Read the model definition and answer for the solid it produces. Units are mm, in the model's axes. A direction names the side the tool comes from. Coordinates: 2 decimals unless noted, no trailing zeros. Order: outer loops, then holes, each group sorted by start corner. A loop starts at its lowest first (then second) coordinate and runs counter-clockwise, first axis right, second up. Notation, with made-up numbers: (-22.5, 3.25) -> (34.5, 3.25) arc R15 cw to (34.5, 12.25) -> close; hole circle Ø11 at (34.25, 55). An arc over 180 degrees is marked (long way). Answer in a Markdown table with one row per item.
from build123d import *

# Parameters (mm, degrees)
SKETCH1_W           = 30
SKETCH1_H           = 10
SKETCH1_R           = 1.75
BOSS_EXTRUDE1_DEPTH = 1
SKETCH2_W           = 30
SKETCH2_H           = 2.5
BOSS_EXTRUDE2_DEPTH = 10
CHAMFER1_SIZE       = 2
CHAMFER1_SIZE2      = 9.409260219


with BuildPart() as part:
    # Sketch1 → Boss-Extrude1 (new body)
    with BuildSketch(Plane.XY):
        Rectangle(SKETCH1_W, SKETCH1_H)
        with Locations((-10, 0.2)):
            Circle(SKETCH1_R, mode=Mode.SUBTRACT)
        with Locations((10, 0.2)):
            Circle(SKETCH1_R, mode=Mode.SUBTRACT)
    extrude(amount=BOSS_EXTRUDE1_DEPTH)

    # Sketch2 → Boss-Extrude2 (add)
    with BuildSketch(Plane.XY):
        with Locations((0, -6.25)):
            Rectangle(SKETCH2_W, SKETCH2_H)
    extrude(amount=BOSS_EXTRUDE2_DEPTH)

    # Chamfer1
    chamfer1_edges = [part.edges().sort_by_distance(p)[0] for p in [
        (0, -7.5, 10),
    ]]
    chamfer1_side = [part.faces().sort_by_distance(p)[0] for p in [
        (0, -6.25, 10),
    ]]
    chamfer(chamfer1_edges, length=CHAMFER1_SIZE, length2=CHAMFER1_SIZE2, reference=chamfer1_side[0])


solid = part.part
Q1. The part is cut by section D-D (y = -2.75). Write down the section's boundary in (x, z), then the cut area to 3 significant figures.
Outcome:
| item | result |
|---|---|
| outline | (-15, 0) -> (15, 0) -> (15, 1) -> (-15, 1) -> close |
| area | 30.0 mm² |
Q2. For a pull along Y with two mould halves and no side action, classify faces 3 (the face through (0, -5, 5)), 4 (the face through (11.669, 0.726, 0.493)), 5 (the face through (0, -1, 0)) as pulls with the +Y half, pulls with the -Y half, needs draft (parallel to the pull), parting line crosses it, or undercut.
Outcome:
| item | result |
|---|---|
| face 3 | pulls with the +Y half |
| face 4 | undercut |
| face 5 | needs draft |
Q3. For faces 1 (the face through (-8.331, 0.726, 0.493)), 2 (the face through (0, 0, 1)), determine the directions among +Z, -Z, +X, -X, +Y, -Y from which every point of the face is accessible in a straight line to the end or side of a thin tool.
Outcome:
| item | result |
|---|---|
| face 1 | +Z, -Z |
| face 2 | +Z, +X, -X, +Y |
Q4. The part is cut by section C-C (x = -5). Write down the section's boundary in (y, z).
Outcome:
| item | result |
|---|---|
| outline | (-7.5, 0) -> (5, 0) -> (5, 1) -> (-5, 1) -> (-5, 10) -> (-5.5, 10) -> (-7.5, 0.59) -> close |
Q5. The part is cut by section A-A (x = -10). Write down the section's boundary in (y, z), then the cut area to 3 significant figures.
Outcome:
| item | result |
|---|---|
| outline | (-7.5, 0) -> (-1.55, 0) -> (-1.55, 1) -> (-5, 1) -> (-5, 10) -> (-5.5, 10) -> (-7.5, 0.59) -> close; (1.95, 0) -> (5, 0) -> (5, 1) -> (1.95, 1) -> close |
| area | 22.1 mm² |
Q6. Given pin 1 (2.5 mm diameter, centred on x = 2, z = 7, fed in from +Y); pin 2 (5 mm diameter, centred on x = 4.5, y = -1, fed in from +Z); pin 3 (6 mm diameter, centred on x = 2, z = 7.5, fed in from -Y), each flat-ended and moving along its own axis, determine where each tip first touches the part or whether it passes through.
Outcome:
| item | result |
|---|---|
| pin 1 | y = -5 |
| pin 2 | z = 1 |
| pin 3 | y = -6.67 |
Q7. The part is cut by section B-B (y = 0.2). Write down the section's boundary in (x, z), then the cut area to 3 significant figures.
Outcome:
| item | result |
|---|---|
| outline | (-15, 0) -> (-11.75, 0) -> (-11.75, 1) -> (-15, 1) -> close; (-8.25, 0) -> (8.25, 0) -> (8.25, 1) -> (-8.25, 1) -> close; (11.75, 0) -> (15, 0) -> (15, 1) -> (11.75, 1) -> close |
| area | 23.0 mm² |
Q8. Consider line 1 (Z direction, x = 12.25, y = 1.25); line 2 (Y direction, x = 10, z = 0.55); line 3 (Y direction, x = -6.25, z = 4). Determine where each line is inside the solid, lowest interval first.
Outcome:
| item | result |
|---|---|
| line 1 | 0 to 1 |
| line 2 | -7.5 to -1.55, 1.95 to 5 |
| line 3 | -6.78 to -5 |
